from build123d import *

# Parameters (mm, degrees)
SKETCH1_R           = 60
BOSS_EXTRUDE1_DEPTH = 1


with BuildPart() as part:
    # Sketch1 → Boss-Extrude1 (new body)
    with BuildSketch(Plane.XY):
        with BuildLine():
            Line((-73.654599313, 60), (-150.505102572, 60))
            ThreePointArc((-150.505102572, 60), (-169.870019303, 50.811388301), (-175, 30))
            Line((-175, 30), (-175, -30))
            ThreePointArc((-175, -30), (-169.870019303, -50.811388301), (-150.505102572, -60))
            Line((-150.505102572, -60), (-73.654599313, -60))
            ThreePointArc((-73.654599313, -60), (0, -95), (73.654599313, -60))
            Line((73.654599313, -60), (150.505102572, -60))
            ThreePointArc((150.505102572, -60), (169.870019303, -50.811388301), (175, -30))
            Line((175, -30), (175, 30))
            ThreePointArc((175, 30), (169.870019303, 50.811388301), (150.505102572, 60))
            Line((150.505102572, 60), (73.654599313, 60))
            ThreePointArc((73.654599313, 60), (0, 95), (-73.654599313, 60))
        make_face()
        Circle(SKETCH1_R, mode=Mode.SUBTRACT)
        with BuildLine():
            Line((-149.327299657, 10), (-99.327299657, 10))
            ThreePointArc((-99.327299657, 10), (-89.327299657, 0), (-99.327299657, -10))
            Line((-99.327299657, -10), (-149.327299657, -10))
            ThreePointArc((-149.327299657, -10), (-159.327299657, 0), (-149.327299657, 10))
        make_face(mode=Mode.SUBTRACT)
        with BuildLine():
            Line((149.327299657, -10), (99.327299657, -10))
            ThreePointArc((99.327299657, -10), (89.327299657, 0), (99.327299657, 10))
            Line((99.327299657, 10), (149.327299657, 10))
            ThreePointArc((149.327299657, 10), (159.327299657, 0), (149.327299657, -10))
        make_face(mode=Mode.SUBTRACT)
    extrude(amount=BOSS_EXTRUDE1_DEPTH)


solid = part.part
Verification items for the finished model (mm, model axes). A direction names the side the tool comes from. Give positions to 0.01 mm unless a question says otherwise; leave off trailing zeros. Loops run counter-clockwise (first coordinate to the right, second up) from the corner with the lowest first, then second, coordinate; pieces in that order, holes last. Notation, with made-up numbers: (71, 43.25) - (130, 43.25) arc R17 ccw to (130, 58.25) - close; hole circle Ø7 at (-10.5, 71). An arc over 180 degrees is marked (long way). Write item = value, one per line. Start each with the question number.
Q1. Cross-section at B-B, the plane x = -105. Enter the section's corners in (y, z), and give its area (3 significant figures).
Q2. Cross-section at D-D, the plane y = 39. Enter the section's corners in (x, z).
Q3. Cross-section at A-A, the plane y = 0. Enter the section's corners in (x, z).
Q4. Thickness scan on line 1 (X direction, y = 3, z = 0.35); line 2 (Y direction, x = 133.5, z = 0.45); line 3 (Y direction, x = -12, z = 0.8). Record the ranges inside material, lowest first.
Q5. Tool access check on faces 1 (the face through (-89.33, 0.22, 0.49)), 2 (the face through (1.18, 94.993, 0.493)). Record the directions out of +Z, -Z, +X, -X, +Y, -Y that give a thin tool (end or side, any length) a straight path to the whole face; none if there is none.
Q6. Cross-section at C-C, the plane z = 0.45. Enter the section's corners in (x, y), and give its area (3 significant figures).
Q7. Depth check by flat-ended pin: P1, Ø12, axis at x = 100, y = -2.5, coming from the -Z side; P2, Ø0.5, axis at x = 119.5, z = 0.5, coming from the +Y side. Enter the tip coordinate at first touch or a pass-through.
Answer key:
q1.outline = (-60, 0) - (-10, 0) - (-10, 1) - (-60, 1) - close; (10, 0) - (60, 0) - (60, 1) - (10, 1) - close
q1.area = 100 mm^2
q2.outline = (-175.18, 0) - (-45.6, 0) - (-45.6, 1) - (-175.18, 1) - close; (45.6, 0) - (175.18, 0) - (175.18, 1) - (45.6, 1) - close
q3.outline = (-175, 0) - (-159.33, 0) - (-159.33, 1) - (-175, 1) - close; (-89.33, 0) - (-60, 0) - (-60, 1) - (-89.33, 1) - close; (60, 0) - (89.33, 0) - (89.33, 1) - (60, 1) - close; (159.33, 0) - (175, 0) - (175, 1) - (159.33, 1) - close
q4.line_1 = -175 to -158.87, -89.79 to -59.92, 59.92 to 89.79, 158.87 to 175
q4.line_2 = -60 to -10, 10 to 60
q4.line_3 = -94.24 to -58.79, 58.79 to 94.24
q5.face_1 = +Z, -Z
q5.face_2 = +Z, -Z, +Y
q6.outline = (-175, -30) arc R25 ccw to (-150.51, -60) - (-73.65, -60) arc R95 ccw to (73.65, -60) - (150.51, -60) arc R25 ccw to (175, -30) - (175, 30) arc R25 ccw to (150.51, 60) - (73.65, 60) arc R95 ccw to (-73.65, 60) - (-150.51, 60) arc R25 ccw to (-175, 30) - close; hole (-149.33, -10) - (-99.33, -10) arc R10 ccw to (-99.33, 10) - (-149.33, 10) arc R10 ccw to start; hole circle Ø120 at (0, 0); hole (99.33, -10) - (149.33, -10) arc R10 ccw to (149.33, 10) - (99.33, 10) arc R10 ccw to start
q6.area = 34,800 mm^2
q7.P1 = through
q7.P2 = 60
